Verification items for the finished model (mm, model axes). A direction names the side the tool comes from. Give positions to 0.01 mm unless a question says otherwise; leave off trailing zeros. Loops run counter-clockwise (first coordinate to the right, second up) from the corner with the lowest first, then second, coordinate; pieces in that order, holes last. Notation, with made-up numbers: M -5,89.25 L 19,89.25 A17 ccw 19,113.25 Z; hole C 63.5,-36.5 d1. An arc over 180 degrees is marked long. Put each result on its own line as item: value. Start each with the question number.
from build123d import *

# Parameters (mm, degrees)
ESQUISSE1_W             = 21
ESQUISSE1_H             = 17
BOSS_EXTRU_1_DEPTH      = 1
BOSS_EXTRU_2_START      = -4
BOSS_EXTRU_2_DEPTH      = 1
ESQUISSE1_4_W           = 21
ESQUISSE1_4_H           = 2.5
BOSS_EXTRU_3_DEPTH      = 4
ENL_V_START             = -1
ESQUISSE1_6_W           = 19.5
ESQUISSE1_6_H           = 2
ENL_V_MAT_EXTRU_1_DEPTH = 2
BOSS_EXTRU_4_START      = -3
BOSS_EXTRU_4_DEPTH      = 13


with BuildPart() as part:
    # Esquisse1 → Boss.-Extru.1 (new body)
    with BuildSketch(Plane.XY):
        Rectangle(ESQUISSE1_W, ESQUISSE1_H)
    extrude(amount=BOSS_EXTRU_1_DEPTH)



with BuildPart() as body_2:
    # Esquisse1_3 → Boss.-Extru.2 (new body)
    with BuildSketch(Plane.XY.offset(BOSS_EXTRU_2_START)):
        Polygon((-10.5, 8.5), (-10.5, -8.5), (10.5, -8.5), (10.5, -3.5), (-1, -3.5), (-1, 3.5), (10.5, 3.5), (10.5, 8.5), align=None)
    extrude(amount=-BOSS_EXTRU_2_DEPTH)


with BuildPart() as part_1:
    add(part.part)

    add(body_2.part)  # Boss.-Extru.3 merges body 2
    # Esquisse1_4 → Boss.-Extru.3 (add)
    with BuildSketch(Plane.XY):
        with Locations((0, 7.25)):
            Rectangle(ESQUISSE1_4_W, ESQUISSE1_4_H)
        with Locations((0, -7.25)):
            Rectangle(ESQUISSE1_4_W, ESQUISSE1_4_H)
    extrude(amount=-BOSS_EXTRU_3_DEPTH)

    # Esquisse1_6 → Enl_v. mat.-Extru.1 (cut)
    with BuildSketch(Plane.XY.offset(ENL_V_START)):
        with Locations((0.75, -7)):
            Rectangle(ESQUISSE1_6_W, ESQUISSE1_6_H)
        with Locations((0.75, 7)):
            Rectangle(ESQUISSE1_6_W, ESQUISSE1_6_H)
    extrude(amount=-ENL_V_MAT_EXTRU_1_DEPTH, mode=Mode.SUBTRACT)

    # Esquisse2 → Boss.-Extru.4 (add)
    with BuildSketch(Plane.ZY.offset(10.5).offset(BOSS_EXTRU_4_START)):
        Polygon((3, 3), (1, 3), (1, -3), (3, -3), (3, -5), (5, -5), (5, -4), (4, -4), (4, -2), (2, -2), (2, 2), (4, 2), (4, 4), (5, 4), (5, 5), (3, 5), align=None)
    extrude(amount=-BOSS_EXTRU_4_DEPTH)


solid = part_1.part
Q1. Cross-section at C-C, the plane y = -4.75. Record the boundary of the cut face in (x, z).
Q2. Scan lines: L1, parallel to Z at x = 1.25, y = -4.5; L2, parallel to Z at x = 3.25, y = -6.5; L3, parallel to Z at x = -7.25, y = 2.75. Record each from-to range of solid material in increasing order.
Q3. Set-up check for faces 1 (the face through (4.7, 3.5, -4.5)), 2 (the face through (1, 8, -2)), 3 (the face through (-1, 3, 4)), 4 (the face through (-1, -5, 4)): record each of +Z, -Z, +X, -X, +Y, -Y from which the full face is reachable in a straight line by a thin tool's end or side.
Q4. Cross-section at A-A, the plane y = -1.75. Record the boundary of the cut face in (x, z).
Q5. Cross-section at D-D, the plane z = 2.5. Record the boundary of the cut face in (x, y).
Q6. Release check for a two-part mould opening along Y. For faces 5 (the face through (-1, 0, -4.5)), 6 (the face through (-1, -3, 2)), 7 (the face through (-1.1, -4.5, 5)), 8 (the face through (-9, 7, -2)) record: pulls with the +Y half, pulls with the -Y half, needs draft (parallel to the pull), parting line crosses it, or undercut.
Q7. Go/stop test with flat-tipped pins: pin 1 (3 mm diameter, centred on y = 2, z = -0.5, fed in from +X); pin 2 (1 mm diameter, centred on x = -2.5, y = -7, fed in from +Z); pin 3 (3 mm diameter, centred on y = 2, z = 3, fed in from +X); pin 4 (1.6 mm diameter, centred on x = 2, z = 4, fed in from -Y). Record where each tip stops, or that it passes through.
Ans:
1. outline: M -10.5,-5 L 10.5,-5 L 10.5,-4 L -10.5,-4 Z; M -10.5,0 L 10.5,0 L 10.5,1 L -10.5,1 Z; M -7.5,3 L 5.5,3 L 5.5,5 L -7.5,5 Z
2. L1: z = -5 to -4, 0 to 1, 3 to 5
2. L2: z = -5 to -3, -1 to 1
2. L3: z = -5 to -4, 0 to 4
3. face 1: -Z, +X
3. face 2: +X
3. face 3: +Z, +X, -X
3. face 4: +Z, +X, -X, -Y
4. outline: M -10.5,-5 L -1,-5 L -1,-4 L -10.5,-4 Z; M -10.5,0 L 10.5,0 L 10.5,1 L 5.5,1 L 5.5,2 L -7.5,2 L -7.5,1 L -10.5,1 Z
5. outline: M -7.5,-3 L 5.5,-3 L 5.5,-2 L -7.5,-2 Z; M -7.5,2 L 5.5,2 L 5.5,3 L -7.5,3 Z
6. face 5: undercut
6. face 6: pulls with the -Y half
6. face 7: needs draft
6. face 8: undercut
7. pin 1: stops at x = 10.5
7. pin 2: stops at z = 1
7. pin 3: stops at x = 5.5
7. pin 4: stops at y = -5
